Read the model definition and answer for the solid it produces. Units are mm, in the model's axes. A direction names the side the tool comes from. Give positions to 0.01 mm unless a question says otherwise; leave off trailing zeros. Order: outer loops, then holes, each group sorted by start corner. A loop starts at its lowest first (then second) coordinate and runs counter-clockwise, first axis right, second up. Notation, with made-up numbers: (37.25, 49) - (83.25, 49) arc R14 ccw to (83.25, 69) - close; hole circle Ø8 at (20, 34.25). An arc over 180 degrees is marked (long way). Use a Markdown table: item, result. Add a question column.
1. For a pull along Z with two mould halves and no side action, classify faces 1 (the cylindrical face through (3, -5, 0)), 2 (the cylindrical face through (3.131, 0.099, -7.502)), 3 (the flat face through (0, 3, 0)), 4 (the cylindrical face through (3.131, 11.172, -7.123)) as released by +Z, released by -Z, zero draft, split by the parting line, or undercut.
2. A cutting plane is placed at A-A on y = 0. Determine the outline of the cut face in (x, z), and give its area (3 significant figures).
3. Flat-ended cylindrical pins translate along their axes: P1, Ø1.9, axis at x = 4, z = -2, coming from the -Y side; P2, Ø3, axis at y = -4.5, z = -2.5, coming from the -X side; P3, Ø2.5, axis at y = 0, z = 9.75, coming from the +X side; P4, Ø1.5, axis at x = 5.5, z = -9.5, coming from the -Y side. Find the tip coordinate at first contact, or state that the pin passes through.
4. A cutting plane is placed at C-C on z = 0. Determine the outline of the cut face in (x, y).
5. A cutting plane is placed at B-B on x = 0.5. Determine the outline of the cut face in (y, z), and give its area (3 significant figures).
6. Which of the six approach directions +Z, -Z, +X, -X, +Y, -Y give full straight-line access (tool end or side, diameter ignored) to faces 5 (the flat face through (3, 2, 0)), 6 (the flat face through (6.35, 3, 0))?
7. A cutting plane is placed at D-D on z = 8.75. Determine the outline of the cut face in (x, y), and give its area (3 significant figures).
8. Consider L1, parallel to Y at x = 2.75, z = 0; L2, parallel to Y at x = 3.25, z = -1.5; L3, parallel to Y at x = 2.25, z = 2.5. Determine where each line is inside the solid, lowest interval first.
```python
from build123d import *

# Parameters (mm, degrees)
SKETCH1_R           = 13.25
SKETCH1_R_2         = 2.25
BOSS_EXTRUDE1_DEPTH = 6.35


with BuildPart() as part:
    # Sketch1 → Boss-Extrude1 (new body)
    with BuildSketch(Plane(origin=(0, 0, 0), x_dir=(0, 0, -1), z_dir=(1, 0, 0))):
        Circle(SKETCH1_R)
        with Locations((-9.75, 0)):
            Circle(SKETCH1_R_2, mode=Mode.SUBTRACT)
        with Locations((0, 9.75)):
            Circle(SKETCH1_R_2, mode=Mode.SUBTRACT)
        with Locations((9.75, 0)):
            Circle(SKETCH1_R_2, mode=Mode.SUBTRACT)
        with Locations((0, -9.75)):
            Circle(SKETCH1_R_2, mode=Mode.SUBTRACT)
        with BuildLine():
            Line((-4.582575695, 2), (4.582575695, 2))
            ThreePointArc((4.582575695, 2), (0, -5), (-4.582575695, 2))
        make_face(mode=Mode.SUBTRACT)
    extrude(amount=BOSS_EXTRUDE1_DEPTH)


solid = part.part
```
Output values:
| question | item | result |
|---|---|---|
| 1 | face 1 | undercut |
| 1 | face 2 | undercut |
| 1 | face 3 | zero draft |
| 1 | face 4 | split by the parting line |
| 2 | outline | (0, -13.25) - (6.35, -13.25) - (6.35, -12) - (0, -12) - close; (0, -7.5) - (6.35, -7.5) - (6.35, -5) - (0, -5) - close; (0, 5) - (6.35, 5) - (6.35, 7.5) - (0, 7.5) - close; (0, 12) - (6.35, 12) - (6.35, 13.25) - (0, 13.25) - close |
| 2 | area | 47.6 mm² |
| 3 | P1 | y = -13.21 |
| 3 | P2 | x = 0 |
| 3 | P3 | through |
| 3 | P4 | y = -9.95 |
| 4 | outline | (0, -13.25) - (6.35, -13.25) - (6.35, -12) - (0, -12) - close; (0, -7.5) - (6.35, -7.5) - (6.35, -5) - (0, -5) - close; (0, 2) - (6.35, 2) - (6.35, 7.5) - (0, 7.5) - close; (0, 12) - (6.35, 12) - (6.35, 13.25) - (0, 13.25) - close |
| 5 | outline | circle Ø26.5 at (0, 0); hole circle Ø4.5 at (-9.75, 0); hole circle Ø4.5 at (0, -9.75); hole circle Ø4.5 at (0, 9.75); hole (2, -4.58) - (2, 4.58) arc R5 ccw (long way) to start; hole circle Ø4.5 at (9.75, 0) |
| 5 | area | 429 mm² |
| 6 | face 5 | +X, -X |
| 6 | face 6 | +Z, -Z, +X, +Y, -Y |
| 7 | outline | (0, -9.95) - (6.35, -9.95) - (6.35, -2.02) - (0, -2.02) - close; (0, 2.02) - (6.35, 2.02) - (6.35, 9.95) - (0, 9.95) - close |
| 7 | area | 101 mm² |
| 8 | L1 | -13.25 to -12, -7.5 to -5, 2 to 7.5, 12 to 13.25 |
| 8 | L2 | -13.16 to -11.43, -8.07 to -4.77, 2 to 8.07, 11.43 to 13.16 |
| 8 | L3 | -13.01 to -4.33, 2 to 13.01 |
